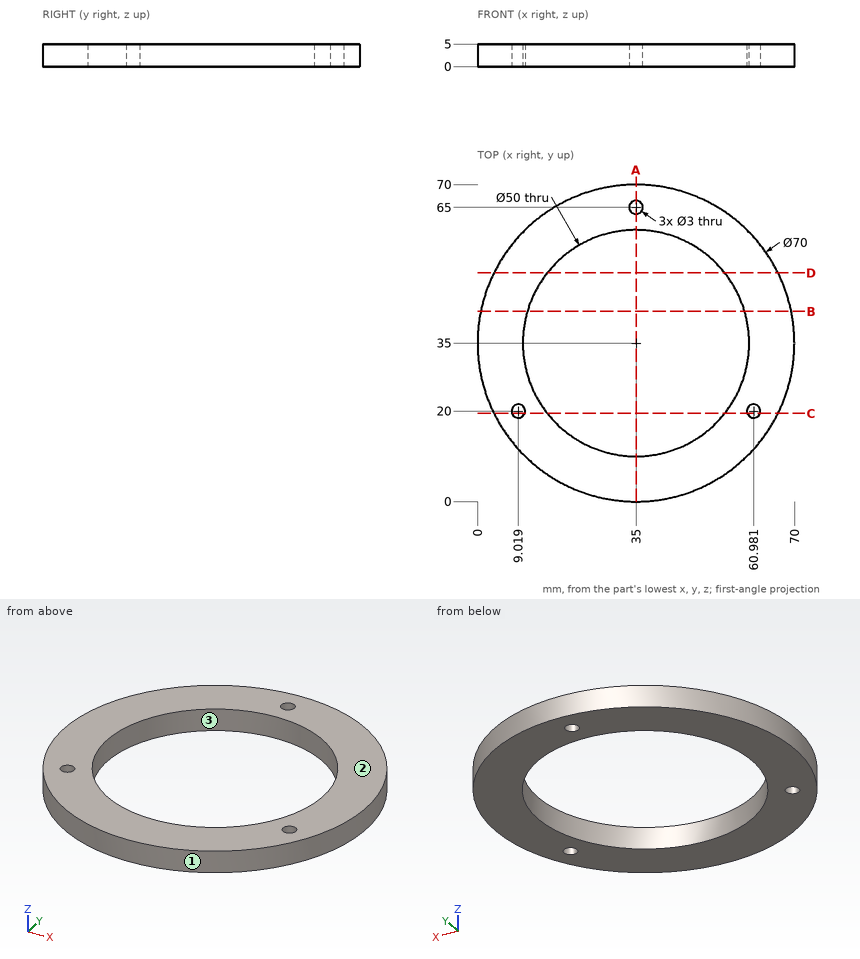
For this review, use the dimensioned drawing (mm, ordinates from the lowest corner) and the shaded views. Give positions to 0.01 mm unless a question says otherwise; leave off trailing zeros. Order: outer loops, then holes, each group sorted by start corner. A loop starts at its lowest first (then second) coordinate and runs counter-clockwise, first axis right, second up.
1) Take a section at A-A (x = 35). Give the boundary of the cut face in (y, z), then the cut area to 3 significant figures.
2) Take a section at B-B (y = 42). Give the boundary of the cut face in (x, z), then the cut area to 3 significant figures.
3) The part is to be moulded in two halves that separate along X. For the marked faces 1, 2 and 3, say which applies: released by +X, released by -X, zero draft, split by the parting line, or undercut.
4) Wall thickness on line 1 (Y direction, x = 35, z = 1.7); line 2 (X direction, y = 20, z = 2.8); line 3 (Y direction, x = 54.5, z = 4.4) (1 decimal): over which ranges is each line inside the solid? List them lowest first.
5) Insertion check: pin 1 (2 mm diameter, centred on y = 45.5, z = 2, fed in from -X); pin 2 (4 mm diameter, centred on x = 18.5, y = 21.5, fed in from +Z); pin 3 (3 mm diameter, centred on y = 13, z = 3.5, fed in from +X); pin 4 (1.5 mm diameter, centred on y = 55, z = 1, fed in from +X). Each pin has a flat end and moves straight along its axis. Give the tip position at first contact, or say it passes through.
6) Take a section at C-C (y = 19.5). Give the boundary of the cut face in (x, z) (1 decimal).
7) Take a section at D-D (y = 50.5). Give the boundary of the cut face in (x, z) (1 decimal), then the cut area to 3 significant figures.
Derived:
1. outline: (0, 0) - (10, 0) - (10, 5) - (0, 5) - close; (60, 0) - (63.5, 0) - (63.5, 5) - (60, 5) - close; (66.5, 0) - (70, 0) - (70, 5) - (66.5, 5) - close
1. area: 85.0 mm2
2. outline: (0.71, 0) - (11, 0) - (11, 5) - (0.71, 5) - close; (59, 0) - (69.29, 0) - (69.29, 5) - (59, 5) - close
2. area: 103 mm2
3. face 1: split by the parting line
3. face 2: zero draft
3. face 3: undercut
4. line 1: y = 0 to 10, 60 to 63.5, 66.5 to 70
4. line 2: x = 3.38 to 7.52, 10.52 to 15, 55 to 59.48, 62.48 to 66.62
4. line 3: y = 5.9 to 19.4, 50.6 to 64.1
5. pin 1: stops at x = 1.31
5. pin 2: passes through
5. pin 3: stops at x = 63.37
5. pin 4: stops at x = 64.23
6. outline: (3.6, 0) - (7.6, 0) - (7.6, 5) - (3.6, 5) - close; (10.4, 0) - (15.4, 0) - (15.4, 5) - (10.4, 5) - close; (54.6, 0) - (59.6, 0) - (59.6, 5) - (54.6, 5) - close; (62.4, 0) - (66.4, 0) - (66.4, 5) - (62.4, 5) - close
7. outline: (3.6, 0) - (15.4, 0) - (15.4, 5) - (3.6, 5) - close; (54.6, 0) - (66.4, 0) - (66.4, 5) - (54.6, 5) - close
7. area: 118 mm2
